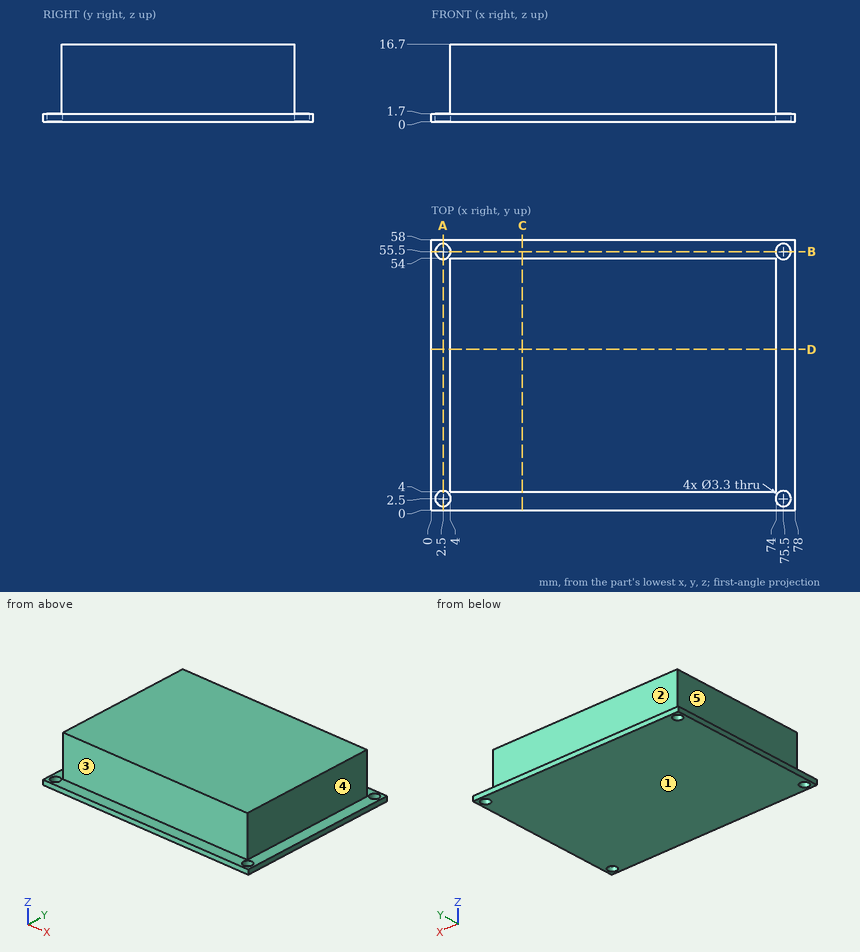
Verification items for this drawing (mm, ordinates from the low corner). A direction names the side the tool comes from. Coordinates: 2 decimals unless noted, no trailing zeros. Write each loop counter-clockwise with the first axis right and the second up, starting at its lowest first coordinate (ties: lowest second). Pieces come first, ordered by that corner, then holes. Notation, with made-up numbers: (85, -38) -> (131, -38) arc R31 cw to (131, -7) -> close; hole circle Ø10 at (-10.75, 42). An arc over 180 degrees is marked (long way). One line per item, written item: value. Start each with the question number.
Q1. Cross-section at B-B on y = 55.5. Enter the section's corners in (x, z), and give its area (3 significant figures).
Q2. Cross-section at A-A on x = 2.5. Enter the section's corners in (y, z), and give its area (3 significant figures).
Q3. Cross-section at C-C on x = 19.5. Enter the section's corners in (y, z).
Q4. Access from +Z, -Z, +X, -X, +Y, -Y to the whole of each face (thin tool, end or side, straight path). Record for the marked faces 1, 2, 3, 4 and 5.
Q5. Cross-section at D-D on y = 34.5. Enter the section's corners in (x, z), and give its area (3 significant figures).
Q6. Thickness scan on L1, parallel to Y at x = 75.5, z = 1.3; L2, parallel to Y at x = 61.5, z = 2.75; L3, parallel to X at y = 53, z = 2.25. Record the ranges inside material, lowest first. Write a range as from..to.
Q7. Go/stop test with flat-tipped pins: P1, Ø4.5, axis at y = 28, z = 10.5, coming from the +X side; P2, Ø4, axis at x = 2.5, y = 2.5, coming from the +Z side; P3, Ø5, axis at x = 35, z = 14.5, coming from the +Y side. Record where each tip stops, or that it passes through.
Checked values:
1. outline: (0, 0) -> (0.85, 0) -> (0.85, 1.7) -> (0, 1.7) -> close; (4.15, 0) -> (73.85, 0) -> (73.85, 1.7) -> (4.15, 1.7) -> close; (77.15, 0) -> (78, 0) -> (78, 1.7) -> (77.15, 1.7) -> close
1. area: 121 mm²
2. outline: (0, 0) -> (0.85, 0) -> (0.85, 1.7) -> (0, 1.7) -> close; (4.15, 0) -> (53.85, 0) -> (53.85, 1.7) -> (4.15, 1.7) -> close; (57.15, 0) -> (58, 0) -> (58, 1.7) -> (57.15, 1.7) -> close
2. area: 87.4 mm²
3. outline: (0, 0) -> (58, 0) -> (58, 1.7) -> (54, 1.7) -> (54, 16.7) -> (4, 16.7) -> (4, 1.7) -> (0, 1.7) -> close
4. face 1: -Z, +X, -X, +Y, -Y
4. face 2: +Z, +X, -X, +Y
4. face 3: +Z, +X, -X, -Y
4. face 4: +Z, +X, +Y, -Y
4. face 5: +Z, -X, +Y, -Y
5. outline: (0, 0) -> (78, 0) -> (78, 1.7) -> (74, 1.7) -> (74, 16.7) -> (4, 16.7) -> (4, 1.7) -> (0, 1.7) -> close
5. area: 1,180 mm²
6. L1: y = 0..0.85, 4.15..53.85, 57.15..58
6. L2: y = 4..54
6. L3: x = 4..74
7. P1: stops at x = 74
7. P2: stops at z = 1.7
7. P3: stops at y = 54
